Read the model definition and answer for the solid it produces. Units are mm, in the model's axes. Face numbers are marked on the shaded views. Round coordinates to 2 decimals unless told otherwise and drop trailing zeros. Loops run counter-clockwise (first coordinate to the right, second up) from the corner with the lowest first, then second, coordinate; pieces in that order, holes last. Notation, with made-up numbers: (-18, 4) - (-9, 4) arc R20 ccw to (-9, 14) - close; hole circle Ø3 at (17.25, 49). An arc over 180 degrees is marked (long way). Use one line per item in the form item = value. Start each with the question number.
```python
from build123d import *

# Parameters (mm, degrees)
SKETCH1_R                    = 15
SKETCH1_R_2                  = 11
BOSS_EXTRUDE1_DEPTH          = 11
BOSS_EXTRUDE2_DEPTH          = 11
F_3_0_3_DIAMETER_HOLE1_D     = 3
F_3_0_3_DIAMETER_HOLE1_DEPTH = 9.098709071
F_3_0_3_DIAMETER_HOLE1_TIP   = 0.901290929


with BuildPart() as part:
    # Sketch1 → Boss-Extrude1 (new body)
    with BuildSketch(Plane(origin=(0, 0, 0), x_dir=(1, 0, 0), z_dir=(0, 1, 0))):
        with Locations(Location((0, 0, 0), (0, 0, 270))):
            Circle(SKETCH1_R)
        with Locations(Location((0, 0, 0), (0, 0, 270))):
            Circle(SKETCH1_R_2, mode=Mode.SUBTRACT)
    extrude(amount=BOSS_EXTRUDE1_DEPTH)

    # Sketch2 → Boss-Extrude2 (add)
    with BuildSketch(Plane(origin=(0, 0, 0), x_dir=(1, 0, 0), z_dir=(0, 1, 0))):
        with BuildLine():
            Line((-22.5, -18), (-14.098155837, 5.122694797))
            ThreePointArc((-14.098155837, 5.122694797), (0, -15), (14.098155837, 5.122694797))
            Line((14.098155837, 5.122694797), (22.5, -18))
            Line((22.5, -18), (-22.5, -18))
        make_face()
    extrude(amount=BOSS_EXTRUDE2_DEPTH)

    # Ø3.0 (3) Diameter Hole1
    with Locations(Plane.XY.offset(18)):
        with Locations((-12.5, 5.5), (12.5, 5.5)):
            Hole(F_3_0_3_DIAMETER_HOLE1_D / 2, depth=F_3_0_3_DIAMETER_HOLE1_DEPTH)
            with Locations((0, 0, -(F_3_0_3_DIAMETER_HOLE1_DEPTH + F_3_0_3_DIAMETER_HOLE1_TIP / 2))):  # 118° drill point
                Cone(0, F_3_0_3_DIAMETER_HOLE1_D / 2, F_3_0_3_DIAMETER_HOLE1_TIP, mode=Mode.SUBTRACT)


solid = part.part
```
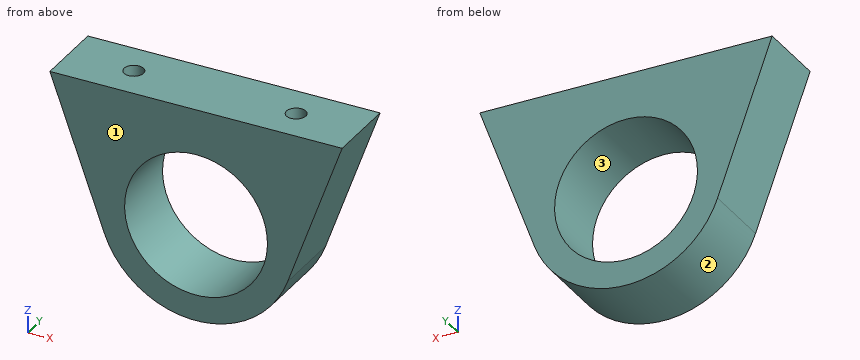
1) Flat-ended cylindrical pins translate along their axes: pin 1 (5 mm diameter, centred on y = 7.5, z = 14, fed in from -X); pin 2 (2 mm diameter, centred on y = 4, z = -7.5, fed in from -X); pin 3 (2 mm diameter, centred on x = 5, y = 7.5, fed in from -Z). Find the tip coordinate at first contact, or state that the pin passes through.
2) Straight lines are drawn through the part: line 1 (Y direction, x = 12.5, z = 13.5); line 2 (X direction, y = 6, z = 13); line 3 (X direction, y = 6.25, z = 0). For each, find the intervals that lie inside material, in ascending order. Write a range as from..to.
3) A cutting plane is placed at C-C on y = 9.25. Write down the section's boundary in (x, z).
4) A cutting plane is placed at A-A on x = 0. Write down the section's boundary in (y, z).
5) Determine the mould class of the marked faces 1, 2 and 3 for opening direction Z: +Z half, -Z half, draft (parallel to the pull), parting line (faces both ways), or undercut.
6) A cutting plane is placed at B-B on z = 0. Write down the section's boundary in (x, y).
7) A cutting plane is placed at D-D on z = 13. Write down the section's boundary in (x, y), plus the area to 3 significant figures.
Checks:
q1.pin_1 = -21.95
q1.pin_2 = -13.52
q1.pin_3 = -14.46
q2.line_1 = 0..4, 7..11
q2.line_2 = -20.68..-13.91, -11.09..11.09, 13.91..20.68
q2.line_3 = -15.96..-11, 11..15.96
q3.outline = (-22.5, 18) - (-14.1, -5.12) arc R15 ccw to (14.1, -5.12) - (22.5, 18) - close; hole circle Ø22 at (0, 0)
q4.outline = (0, -15) - (11, -15) - (11, -11) - (0, -11) - close; (0, 11) - (11, 11) - (11, 18) - (0, 18) - close
q5.face_1 = draft
q5.face_2 = -Z half
q5.face_3 = undercut
q6.outline = (-15.96, 0) - (-11, 0) - (-11, 11) - (-15.96, 11) - close; (11, 0) - (15.96, 0) - (15.96, 11) - (11, 11) - close
q7.outline = (-20.68, 0) - (20.68, 0) - (20.68, 11) - (-20.68, 11) - close; hole circle Ø3 at (-12.5, 5.5); hole circle Ø3 at (12.5, 5.5)
q7.area = 441 mm²
